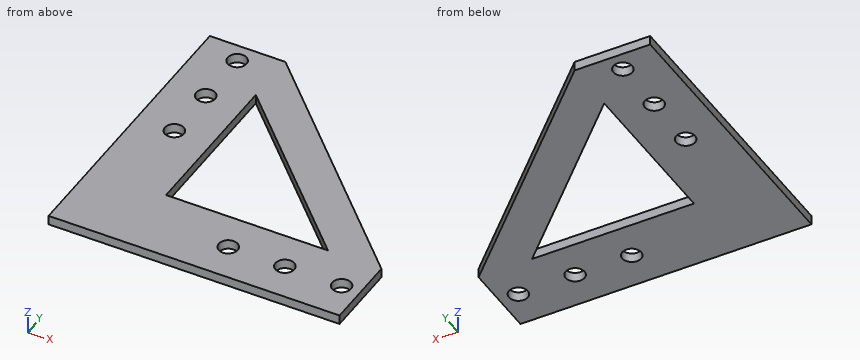
```python
from build123d import *

# Parameters (mm, degrees)
BOSS_EXTRUDE1_DEPTH = 3.175
SKETCH2_R           = 3.175
CUT_EXTRUDE1_DEPTH  = 139.332385308


with BuildPart() as part:
    # Sketch1 → Boss-Extrude1 (new body)
    with BuildSketch(Plane.XY):
        Polygon((25.4, 97.79), (97.79, 25.4), (97.79, 0), (0, 0), (0, 97.79), align=None)
        Polygon((25.4, 25.4), (25.4, 79.829487758), (79.829487758, 25.4), align=None, mode=Mode.SUBTRACT)
    extrude(amount=BOSS_EXTRUDE1_DEPTH)

    # Sketch2 → Cut-Extrude1 (cut, through all)
    with BuildSketch(Plane.XY.offset(3.175)):
        with Locations((53.34, 12.7)):
            Circle(SKETCH2_R)
        with Locations((72.39, 12.7)):
            Circle(SKETCH2_R)
        with Locations((12.7, 53.34)):
            Circle(SKETCH2_R)
        with Locations((12.7, 72.39)):
            Circle(SKETCH2_R)
        with Locations((12.7, 91.44)):
            Circle(SKETCH2_R)
        with Locations((91.44, 12.7)):
            Circle(SKETCH2_R)
    extrude(amount=-CUT_EXTRUDE1_DEPTH, mode=Mode.SUBTRACT)


solid = part.part
```
Can you work these out from the model? Positions are in its coordinate system, mm. Coordinates: 2 decimals unless noted, no trailing zeros. Order: outer loops, then holes, each group sorted by start corner. A loop starts at its lowest first (then second) coordinate and runs counter-clockwise, first axis right, second up.
1. I need wall thicknesses on line 1 (Y direction, x = 12.7, z = 2) (3 decimals); line 2 (Y direction, x = 51, z = 2.4); line 3 (Y direction, x = 15, z = 1.65). Which ranges of each line are inside material? Lowest first, please.
2. If we section it at B-B (y = 91.44): Please give me the cut outline in (x, z) (3 decimals).
3. If we section it at C-C (z = 2.05): Please give me the cut outline in (x, y) (3 decimals), then the cut area to 3 significant figures.
4. If we section it at A-A (x = 12.7): Please give me the cut outline in (y, z) (3 decimals).
5. If we section it at D-D (x = 72.39): Please give me the cut outline in (y, z) (3 decimals), then the cut area to 3 significant figures.
Entries:
1. line 1: y = 0 to 50.165, 56.515 to 69.215, 75.565 to 88.265, 94.615 to 97.79
1. line 2: y = 0 to 10.55, 14.85 to 25.4, 54.23 to 72.19
1. line 3: y = 0 to 51.15, 55.53 to 70.2, 74.58 to 89.25, 93.63 to 97.79
2. outline: (0, 0) - (9.525, 0) - (9.525, 3.175) - (0, 3.175) - close; (15.875, 0) - (31.75, 0) - (31.75, 3.175) - (15.875, 3.175) - close
3. outline: (0, 0) - (97.79, 0) - (97.79, 25.4) - (25.4, 97.79) - (0, 97.79) - close; hole circle Ø6.35 at (12.7, 53.34); hole circle Ø6.35 at (12.7, 72.39); hole circle Ø6.35 at (12.7, 91.44); hole (25.4, 25.4) - (79.829, 25.4) - (25.4, 79.829) - close; hole circle Ø6.35 at (53.34, 12.7); hole circle Ø6.35 at (72.39, 12.7); hole circle Ø6.35 at (91.44, 12.7)
3. area: 5,270 mm2
4. outline: (0, 0) - (50.165, 0) - (50.165, 3.175) - (0, 3.175) - close; (56.515, 0) - (69.215, 0) - (69.215, 3.175) - (56.515, 3.175) - close; (75.565, 0) - (88.265, 0) - (88.265, 3.175) - (75.565, 3.175) - close; (94.615, 0) - (97.79, 0) - (97.79, 3.175) - (94.615, 3.175) - close
5. outline: (0, 0) - (9.525, 0) - (9.525, 3.175) - (0, 3.175) - close; (15.875, 0) - (25.4, 0) - (25.4, 3.175) - (15.875, 3.175) - close; (32.839, 0) - (50.8, 0) - (50.8, 3.175) - (32.839, 3.175) - close
5. area: 118 mm2
